from build123d import *

# Parameters (mm, degrees)
F0_R     = 50.8
F0_R_2   = 5.1562
F0_W     = 19.05
F0_H     = 19.05
F1_DEPTH = 12.7
F2_R     = 25.4
F3_DEPTH = 3.175


with BuildPart() as f1:
    # F0 (on Front) → F1 (new body)
    with BuildSketch(Plane.XZ):
        Circle(F0_R)
        with Locations((0, -41.275)):
            Circle(F0_R_2, mode=Mode.SUBTRACT)
        with Locations((-41.275, 0)):
            Circle(F0_R_2, mode=Mode.SUBTRACT)
        Rectangle(F0_W, F0_H, mode=Mode.SUBTRACT)
        with Locations((41.275, 0)):
            Circle(F0_R_2, mode=Mode.SUBTRACT)
        with Locations((0, 41.275)):
            Circle(F0_R_2, mode=Mode.SUBTRACT)
    extrude(amount=F1_DEPTH)

    # F2 (on Front) → F3 (cut)
    with BuildSketch(Plane.XZ):
        Circle(F2_R)
    extrude(amount=F3_DEPTH, mode=Mode.SUBTRACT)


solid = f1.part
CAD build for the part. Positions are in the model's coordinates, mm. A direction names the side the tool comes from. Round coordinates to 2 decimals unless told otherwise and drop trailing zeros. Loops run counter-clockwise (first coordinate to the right, second up) from the corner with the lowest first, then second, coordinate; pieces in that order, holes last.
(1) Cut at C-C (x = 39). Give the cut face in (y, z).
(2) Cut at A-A (z = 0). Give the cut face in (x, y) (3 decimals).
(3) Drop flat-ended pins along their axis: pin 1 (1.5 mm diameter, centred on x = 22, y = -2.5, fed in from -Z); pin 2 (12 mm diameter, centred on x = -41.275, z = 0, fed in from +Y); pin 3 (12 mm diameter, centred on x = 7, z = 10, fed in from +Y) (3 decimals); pin 4 (5 mm diameter, centred on x = -4, y = -6, fed in from +Z). Give the stop position or say it passes through.
(4) Which spindle directions (+Z, -Z, +X, -X, +Y, -Y) get a long thin tool onto all of the face, cutting with end or side? Do faces 1 (the flat face through (11, -12.7, 1)), 2 (the flat face through (11, -3.175, 0)), 3 (the flat face through (0, -8, 9.525)). Say none if no direction does.
(5) Two-plate mould, pull along Z, no slides. Class faces 4 (the flat face through (-23.3, 0, -10.6)), 5 (the cylindrical face through (-11.012, -6.261, -49.592)), 6 (the cylindrical face through (-5.506, -1.565, -24.796)): +Z half, -Z half, draft (parallel to the pull), parting line (faces both ways), or undercut.
(6) Cut at B-B (x = 0). Give the cut face in (y, z) (3 decimals), plus the area to 3 significant figures.
(7) Cut at D-D (y = -6). Give the cut face in (x, z) (3 decimals), plus the area to 3 significant figures.
(8) Wall check: line 1 along Z through (x, y) = (0, -2.4); line 2 along Z through (x, y) = (0, -4.5) (3 decimals); line 3 along X through (y, z) = (-0.75, 4). Give the ranges that are in metal, low to high.
Findings below:
1. outline: (-12.7, -32.55) - (0, -32.55) - (0, -4.63) - (-12.7, -4.63) - close; (-12.7, 4.63) - (0, 4.63) - (0, 32.55) - (-12.7, 32.55) - close
2. outline: (-50.8, -12.7) - (-46.431, -12.7) - (-46.431, 0) - (-50.8, 0) - close; (-36.119, -12.7) - (-9.525, -12.7) - (-9.525, -3.175) - (-25.4, -3.175) - (-25.4, 0) - (-36.119, 0) - close; (9.525, -12.7) - (36.119, -12.7) - (36.119, 0) - (25.4, 0) - (25.4, -3.175) - (9.525, -3.175) - close; (46.431, -12.7) - (50.8, -12.7) - (50.8, 0) - (46.431, 0) - close
3. pin 1: stops at z = -46.14
3. pin 2: stops at y = 0
3. pin 3: stops at y = -3.175
3. pin 4: stops at z = 50.78
4. face 1: +Z, -Z, +X, -X, -Y
4. face 2: +Y
4. face 3: +Y, -Y
5. face 4: draft
5. face 5: parting line
5. face 6: undercut
6. outline: (-12.7, -50.8) - (0, -50.8) - (0, -46.431) - (-12.7, -46.431) - close; (-12.7, -36.119) - (0, -36.119) - (0, -25.4) - (-3.175, -25.4) - (-3.175, -9.525) - (-12.7, -9.525) - close; (-12.7, 9.525) - (-3.175, 9.525) - (-3.175, 25.4) - (0, 25.4) - (0, 36.119) - (-12.7, 36.119) - close; (-12.7, 46.431) - (0, 46.431) - (0, 50.8) - (-12.7, 50.8) - close
6. area: 686 mm2
7. outline: circle Ø101.6 at (0, 0); hole circle Ø10.312 at (-41.275, 0); hole (-9.525, -9.525) - (9.525, -9.525) - (9.525, 9.525) - (-9.525, 9.525) - close; hole circle Ø10.312 at (0, -41.275); hole circle Ø10.312 at (0, 41.275); hole circle Ø10.312 at (41.275, 0)
7. area: 7,410 mm2
8. line 1: z = -50.8 to -46.43, -36.12 to -25.4, 25.4 to 36.12, 46.43 to 50.8
8. line 2: z = -50.8 to -46.431, -36.119 to -9.525, 9.525 to 36.119, 46.431 to 50.8
8. line 3: x = -50.64 to -44.53, -38.02 to -25.08, 25.08 to 38.02, 44.53 to 50.64
